Here's the drawing with two shaded views (mm, measured from the low corner). I have some questions. Round coordinates to 2 decimals unless told otherwise and drop trailing zeros. Order: outer loops, then holes, each group sorted by start corner. A loop starts at its lowest first (then second) coordinate and runs counter-clockwise, first axis right, second up. Notation, with made-up numbers: (61.5, 29.25) -> (66.5, 29.25) arc R23 cw to (66.5, 38.25) -> close; hole circle Ø6 at (-29.75, 54.5). An arc over 180 degrees is marked (long way). One line per question, with ' | ' between items.
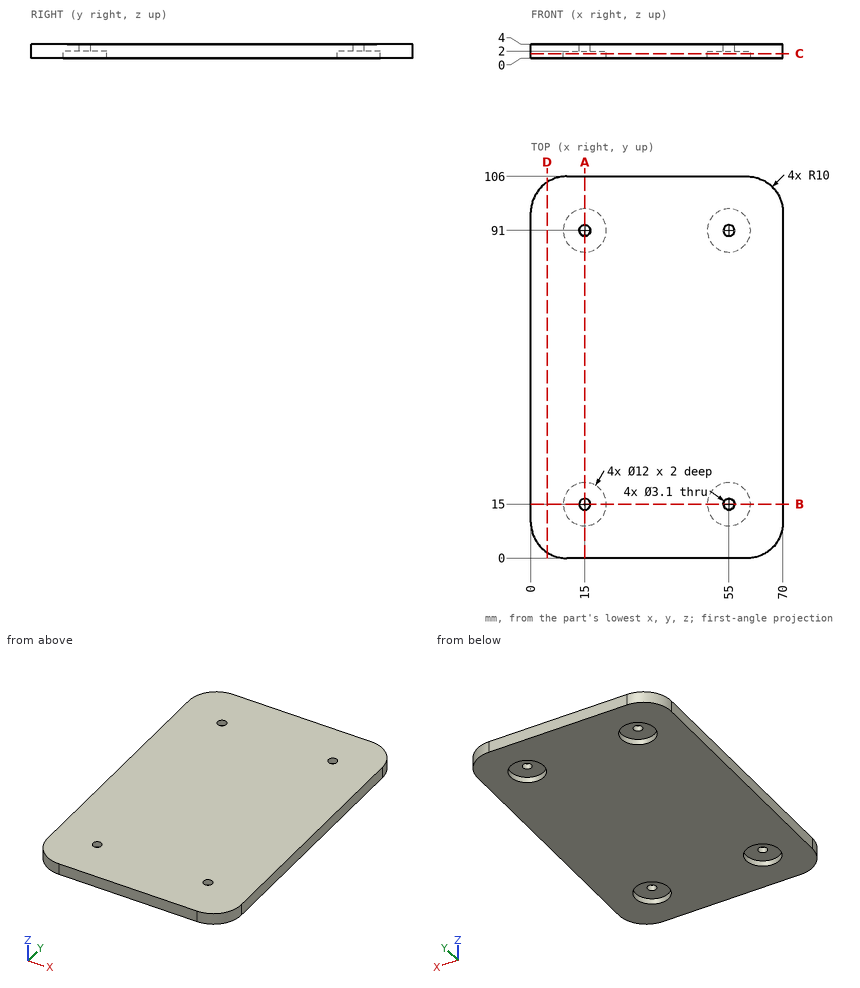
1. I'm going to push a flat-ended pin straight in: pin 1 (5 mm diameter, centred on x = 15, y = 91, fed in from -Z). Where does the tip first touch, or does it pass through?
From the geometry:
pin 1: stops at z = 2
2. I want a section at A-A on x = 15. List the corners of the cut face in (y, z) for me.
From the geometry:
outline: (0, 0) -> (9, 0) -> (9, 2) -> (13.45, 2) -> (13.45, 4) -> (0, 4) -> close; (16.55, 2) -> (21, 2) -> (21, 0) -> (85, 0) -> (85, 2) -> (89.45, 2) -> (89.45, 4) -> (16.55, 4) -> close; (92.55, 2) -> (97, 2) -> (97, 0) -> (106, 0) -> (106, 4) -> (92.55, 4) -> close
3. I want a section at B-B on y = 15. List the corners of the cut face in (x, z) for me, and give its area (3 significant figures).
From the geometry:
outline: (0, 0) -> (9, 0) -> (9, 2) -> (13.45, 2) -> (13.45, 4) -> (0, 4) -> close; (16.55, 2) -> (21, 2) -> (21, 0) -> (49, 0) -> (49, 2) -> (53.45, 2) -> (53.45, 4) -> (16.55, 4) -> close; (56.55, 2) -> (61, 2) -> (61, 0) -> (70, 0) -> (70, 4) -> (56.55, 4) -> close | area: 220 mm²
4. I need wall thicknesses on probe 1 along X at (y, z) = (15, 1.4); probe 2 along Y at (x, z) = (15.5, 1.9); probe 3 along X at (y, z) = (10, 1.55). Which ranges of each line are inside material? Lowest first, please.
From the geometry:
probe 1: x = 0 to 9, 21 to 49, 61 to 70 | probe 2: y = 0 to 9.02, 20.98 to 85.02, 96.98 to 106 | probe 3: x = 0 to 11.68, 18.32 to 51.68, 58.32 to 70
5. I want a section at D-D on x = 4.5. List the corners of the cut face in (y, z) for me.
From the geometry:
outline: (1.65, 0) -> (104.35, 0) -> (104.35, 4) -> (1.65, 4) -> close
6. I want a section at C-C on z = 1.35. List the corners of the cut face in (x, y) for me.
From the geometry:
outline: (0, 10) arc R10 ccw to (10, 0) -> (60, 0) arc R10 ccw to (70, 10) -> (70, 96) arc R10 ccw to (60, 106) -> (10, 106) arc R10 ccw to (0, 96) -> close; hole circle Ø12 at (15, 15); hole circle Ø12 at (15, 91); hole circle Ø12 at (55, 15); hole circle Ø12 at (55, 91)
